Autodesk Inventor part; units mm, degrees
ref_plane "YZ Plane" through (0, 0, 0) normal (1, 0, 0) x (0, 1, 0)
ref_plane "XZ Plane" through (0, 0, 0) normal (0, 1, 0) x (-1, 0, 0)
ref_plane "XY Plane" through (0, 0, 0) normal (0, 0, 1) x (1, 0, 0)
sketch "Sketch1" plane through (0, 0, 0) normal (0, 0, 1) x (1, 0, 0)
  arc A0 (-0.4474, 4.2264) -> (0.4474, 4.2264) centre (0, 0) ccw
  line L0 (10, 10) -> (10, -23)
  line L1 (10, -23) -> (-10, -23)
  line L2 (-10, -23) -> (-10, 10)
  line L3 (-0.4474, 4.2264) -> (-0.4474, 10)
  line L4 (0.4474, 4.2264) -> (0.4474, 10)
  line L5 (-10, 10) -> (-0.4474, 10)
  line L6 (0.4474, 10) -> (10, 10)
  dimension "d2" = 8.5
  dimension "d3" = 20
  dimension "d7" = 23
  dimension "d43" = 10
  dimension "d44" = 10
extrude "Extrusion1" add sketch "Sketch1" along normal blind 15
sketch "Sketch2" plane through (-10, -23, 0) normal (0, -1, 0) x (1, 0, 0)
  line L0 (0, 0) -> (0, 15)
  line L1 (20, 0) -> (20, 15)
  line L2 (0, 0) -> (20, 15)
  line L3 (-10, 15) -> (30, 15)
  line L4 (30, 15) -> (30, 0)
  line L5 (30, 0) -> (-10, 0)
  line L6 (-10, 0) -> (-10, 15)
  line L7 (-10, 15) -> (30, 0) construction
  line L8 (30, 15) -> (-10, 0) construction
  point P0 (10, 0)
  point P1 (10, 7.5)
  dimension "d13" = 40
  dimension "d17" = 15
extrude "Extrusion2" add sketch "Sketch2" along normal blind 6
sketch "Sketch3" plane through (-10, -29, 0) normal (0, -1, 0) x (1, 0, 0)
  line L0 (-10, 10.5) -> (30, 10.5)
  line L1 (-10, 4.5) -> (30, 4.5)
  line L2 (-10, 4.5) -> (-10, 10.5)
  line L3 (-10, 0) -> (-10, 15)
  line L4 (30, 10.5) -> (30, 4.5)
  line L5 (30, 0) -> (30, 15)
  point P0 (10, 0)
extrude "Extrusion3" add sketch "Sketch3" along normal blind 1.5
sketch "Sketch4" plane through (-10, -30.5, 0) normal (0, -1, 0) x (1, 0, 0)
  line L0 (30, 4.5) -> (-10, 4.5)
  line L1 (-10, 10.5) -> (30, 10.5)
  line L2 (-10, 10.5) -> (-10, 4.5)
  line L3 (-10, 7.5) -> (-5, 7.5)
  line L4 (30, 15) -> (30, 0)
  line L5 (30, 7.5) -> (25, 7.5)
  point P0 (10, 0)
  dimension "d22" = 5
  dimension "d23" = 5
hole "Hole1" at (-15, -30.5, 7.5) at (15, -30.5, 7.5) direction (0, 1, 0) diameter 5.5 end through all counterbore diameter 10 counterbore depth 1.5
sketch "Sketch5" plane through (10, 10, 15) normal (1, 0, 0) x (0, 0, -1)
  line L0 (15, 0) -> (0, 0)
  line L1 (7.5, 0) -> (7.5, -3)
  point P0 (15, -10)
  dimension "d35" = 3
hole "Hole2" at (10, 7, 7.5) direction (-1, 0, 0) diameter 4 end through all
properties part number "Suporte Eixos 8mm"
Could you check a few things on this model? Use its own coordinates, in mm. A direction names the side the tool comes from. Coordinates: 2 decimals unless noted, no trailing zeros. Order: outer loops, then holes, each group sorted by start corner. A loop starts at its lowest first (then second) coordinate and runs counter-clockwise, first axis right, second up. Notation, with made-up numbers: M 71,-23 L 78,-23 A21 cw 78,-9 Z; hole C 26.25,32 d8. An arc over 180 degrees is marked long. Use a Markdown table: item, result. Add a question column.
Q1. If I drill on L1, parallel to X at y = -24.95, z = 7.5; L2, parallel to X at y = -25, z = 5; L3, parallel to Y at x = -1.5, z = 5.75, over which ranges is the centre line in solid material (lowest first)?
Q2. Which directions (+Z, -Z, +X, -X, +Y, -Y) give clear straight access to the entire face, cutting with the end or side of a thin tool? Please do faces 1 (the flat face through (-10, -7, 7)), 2 (the flat face through (0, -30, 10.5)), 3 (the flat face through (0, -14, 15)), 4 (the flat face through (-19.5, -29.7, 4.5)), 5 (the flat face through (5, 10, 7)).
Q3. I want a section at B-B on y = 7. List the corners of the cut face in (x, z) for me.
Q4. I want a section at C-C on z = 11.25. List the corners of the cut face in (x, y) for me.
Q5. We'd pull the mould along Y, two halves only. Please class faces 6 (the cylindrical face through (-5.291, 6.912, 9.498)), 7 (the flat face through (10, -6, 7)), 8 (the flat face through (-19.7, -30.5, 5.2)): pulls with the +Y half, pulls with the -Y half, needs draft (parallel to the pull), parting line crosses it, or undercut.
Q6. I'm going to push flat-ended pins straight in: pin 1 (3 mm diameter, centred on y = 6.5, z = 6, fed in from -X); pin 2 (7.5 mm diameter, centred on y = 0, z = 6, fed in from +X); pin 3 (8 mm diameter, centred on x = 15.5, z = 6.5, fed in from +Y). Where does each tip first touch, or does it pass through?
Q7. I want a section at A-A on x = 15. List the corners of the cut face in (y, z) for me.
Q8. I want a section at D-D on x = -2. List the corners of the cut face in (y, z) for me, then the cut area to 3 significant figures.
Checked values:
| question | item | result |
|---|---|---|
| 1 | L1 | -20 to -17.75, -12.25 to 12.25, 17.75 to 20 |
| 1 | L2 | -20 to -16.15, -13.85 to 13.85, 16.15 to 20 |
| 1 | L3 | -30.5 to -3.98, 3.98 to 6.03, 7.97 to 10 |
| 2 | face 1 | +Z, -Z, -X, +Y |
| 2 | face 2 | +Z, +X, -X, -Y |
| 2 | face 3 | +Z, +X, -X, +Y, -Y |
| 2 | face 4 | -Z, +X, -X, -Y |
| 2 | face 5 | +Z, -Z, +X, -X, +Y |
| 3 | outline | M -10,0 L -0.45,0 L -0.45,5.5 L -10,5.5 Z; M -10,9.5 L -0.45,9.5 L -0.45,15 L -10,15 Z; M 0.45,0 L 10,0 L 10,5.5 L 0.45,5.5 Z; M 0.45,9.5 L 10,9.5 L 10,15 L 0.45,15 Z |
| 4 | outline | M -20,-29 L 20,-29 L 20,-23 L 10,-23 L 10,10 L 0.45,10 L 0.45,4.23 A4.25 cw long -0.45,4.23 L -0.45,10 L -10,10 L -10,-23 L -20,-23 Z |
| 5 | face 6 | undercut |
| 5 | face 7 | needs draft |
| 5 | face 8 | pulls with the -Y half |
| 6 | pin 1 | x = -10 |
| 6 | pin 2 | x = 10 |
| 6 | pin 3 | y = -23 |
| 7 | outline | M -29,0 L -23,0 L -23,4.75 L -29,4.75 Z; M -29,10.25 L -23,10.25 L -23,15 L -29,15 Z |
| 8 | outline | M -30.5,4.5 L -29,4.5 L -29,0 L -3.75,0 L -3.75,15 L -29,15 L -29,10.5 L -30.5,10.5 Z; M 3.75,0 L 10,0 L 10,15 L 3.75,15 Z; hole C 7,7.5 d4 |
| 8 | area | 469 mm² |
